from build123d import *

# Parameters (mm, degrees)
CYLINDER117_R     = 1.2
CYLINDER117_DEPTH = 100
FILLET009_R       = 1
FILLET010_R       = 1


with BuildPart() as obj1:
    # Cylinder117 → Cylinder117 (new body)
    with BuildSketch(Plane.XY.offset(-50)):
        Circle(CYLINDER117_R)
    extrude(amount=CYLINDER117_DEPTH)


with BuildPart() as obj2:
    # Cone009 → Cone009 (revolve)
    with BuildSketch(Plane(origin=(0, 0, -3), x_dir=(1, 0, 0), z_dir=(0, -1, 0))):
        Polygon((0, 0), (1.2, 0), (2, 3), (0, 3), align=None)
    revolve(axis=Axis((0, 0, -3), (0, 0, 1)))


with BuildPart() as syringe_tip_hole_fusion001:
    # Cone005 → Cone005 (revolve)
    with BuildSketch(Plane.XZ):
        Polygon((0, 0), (2, 0), (2.2, 6.6), (0, 6.6), align=None)
    revolve(axis=Axis((0, 0, 0), (0, 0, 1)))

    # Fusion019: union obj1, obj2
    add(obj1.part)
    add(obj2.part)


with BuildPart() as obj3:
    # Cone008 → Cone008 (revolve)
    with BuildSketch(Plane(origin=(0, 0, -3), x_dir=(1, 0, 0), z_dir=(0, -1, 0))):
        Polygon((0, 0), (2.8, 0), (4, 3), (0, 3), align=None)
    revolve(axis=Axis((0, 0, -3), (0, 0, 1)))


with BuildPart() as obj4:
    # Cone007 → Cone007 (revolve)
    with BuildSketch(Plane(origin=(0, 0, -11), x_dir=(1, 0, 0), z_dir=(0, -1, 0))):
        Polygon((0, 0), (2.5, 0), (2.8, 8), (0, 8), align=None)
    revolve(axis=Axis((0, 0, -11), (0, 0, 1)))

    # Fillet009
    fillet009_edges = [obj4.edges().sort_by_distance(p)[0] for p in [
        (-2.5, 0, -11),
    ]]
    fillet(fillet009_edges, radius=FILLET009_R)


with BuildPart() as syringe_tip_cut_fillet001:
    # Cone006 → Cone006 (revolve)
    with BuildSketch(Plane.XZ):
        Polygon((0, 0), (4, 0), (4.2, 6.6), (0, 6.6), align=None)
    revolve(axis=Axis((0, 0, 0), (0, 0, 1)))

    # Fusion018: union obj3, obj4
    add(obj3.part)
    add(obj4.part)

    # Cut013: cut syringe tip hole fusion001
    add(syringe_tip_hole_fusion001.part, mode=Mode.SUBTRACT)

    # Fillet010
    fillet010_edges = [syringe_tip_cut_fillet001.edges().sort_by_distance(p)[0] for p in [
        (-2.2, 0, 6.6),
    ]]
    fillet(fillet010_edges, radius=FILLET010_R)


solid = syringe_tip_cut_fillet001.part
Geometry check sheet. Reference: the model listing, model coordinates, mm. A direction names the side the tool comes from. Round coordinates to 2 decimals unless told otherwise and drop trailing zeros. Order: outer loops, then holes, each group sorted by start corner. A loop starts at its lowest first (then second) coordinate and runs counter-clockwise, first axis right, second up. Notation, with made-up numbers: M 0,-12 L 49,-12 A16 cw 49,13 Z; hole C 89,5.25 d1. An arc over 180 degrees is marked long. Answer in a Markdown table with one row per item. Add a question column.
Item 1: Material ranges on L1, parallel to Y at x = 0, z = -9 (3 decimals); L2, parallel to Y at x = 1.5, z = -1; L3, parallel to X at y = 0, z = -5 (3 decimals), recorded low to high. Write a range as [from, to].
Item 2: Sectioned sample at A-A, the plane y = 0. Enter the section's corners in (x, z).
Item 3: Draft check along X on faces 1 (the face through (-0.197, 1.504, -1.812)), 2 (the face through (-0.6, -2.6, -6.5)), 3 (the face through (-2, 3, 6.6)). Enter one of: released by +X, released by -X, zero draft, split by the parting line, or undercut.
Item 4: Sectioned sample at C-C, the plane z = -1.5. Enter the section's corners in (x, y), plus the area to 3 significant figures.
Item 5: Sectioned sample at D-D, the plane z = -3.5. Enter the section's corners in (x, y), plus the area to 3 significant figures.
Item 6: Set-up check for faces 4 (the face through (-0.9, -4, 3.3)), 5 (the face through (-1.656, -1.27, 2.855)), 6 (the face through (0.65, 1.01, -7.06)): record each of +Z, -Z, +X, -X, +Y, -Y from which the full face is reachable in a straight line by a thin tool's end or side.
Item 7: Depth check by flat-ended pin: pin 1 Ø1.5 at (y, z) = (-1, -8) entering from -X; pin 2 Ø4 at (x, z) = (3, 1) entering from -Y; pin 3 Ø3 at (x, z) = (0.5, -3.5) entering from -Y; pin 4 Ø4 at (x, y) = (0, 3) entering from -Z. Enter the tip coordinate at first touch or a pass-through.
Filled in:
| question | item | result |
|---|---|---|
| 1 | L1 | y = [-2.575, -1.2], [1.2, 2.575] |
| 1 | L2 | y = [-3.27, -0.87], [0.87, 3.27] |
| 1 | L3 | x = [-2.725, -1.2], [1.2, 2.725] |
| 2 | outline | M -4.2,6.6 L -4,0 L -2.8,-3 L -2.54,-10.04 A1 ccw -1.54,-11 L -1.2,-11 L -1.2,-3 L -2,0 L -2.17,5.63 A1 ccw -3.17,6.6 Z; M 1.2,-11 L 1.54,-11 A1 ccw 2.54,-10.04 L 2.8,-3 L 4,0 L 4.2,6.6 L 3.17,6.6 A1 ccw 2.17,5.63 L 2,0 L 1.2,-3 Z |
| 3 | face 1 | undercut |
| 3 | face 2 | split by the parting line |
| 3 | face 3 | zero draft |
| 4 | outline | C 0,0 d6.8; hole C 0,0 d3.2 |
| 4 | area | 28.3 mm² |
| 5 | outline | C 0,0 d5.56; hole C 0,0 d2.4 |
| 5 | area | 19.8 mm² |
| 6 | face 4 | -Z |
| 6 | face 5 | +Z |
| 6 | face 6 | +Z, -Z |
| 7 | pin 1 | stops at x = -2.61 |
| 7 | pin 2 | stops at y = -3.91 |
| 7 | pin 3 | stops at y = -3.18 |
| 7 | pin 4 | stops at z = -11 |
